from build123d import *

# Parameters (mm, degrees)
F0_W     = 44
F0_H     = 55
F2_R     = 20
F3_DEPTH = 133.830428
F4_W     = 29.281278
F4_H     = 21.154624
F5_DEPTH = 25


with BuildPart() as f1:
    # F0 (on Front) → F1 (revolve)
    with BuildSketch(Plane.XZ):
        with Locations((-22, 27.5)):
            Rectangle(F0_W, F0_H)
    revolve(axis=Axis((0, 0, 27.5), (0, 0, -1)))

    # F2 (on face) → F3 (cut)
    with BuildSketch(Plane(origin=(0, 0, 0), x_dir=(1, 0, 0), z_dir=(0, 0, -1))):
        with Locations((0, -15.39881)):
            Circle(F2_R)
    extrude(amount=-F3_DEPTH, mode=Mode.SUBTRACT)

    # F4 (on face) → F5 (cut)
    with BuildSketch(Plane.XY.offset(55)):
        with Locations((6.999669, -21.173684)):
            Rectangle(F4_W, F4_H)
    extrude(amount=-F5_DEPTH, mode=Mode.SUBTRACT)


solid = f1.part
Geometry check sheet. Reference: the model listing, model coordinates, mm. A direction names the side the tool comes from. Round coordinates to 2 decimals unless told otherwise and drop trailing zeros. Write each loop counter-clockwise with the first axis right and the second up, starting at its lowest first coordinate (ties: lowest second). Pieces come first, ordered by that corner, then holes. Notation, with made-up numbers: (64.25, -11.75) -> (82.25, -11.75) arc R22 ccw to (82.25, 11.25) -> close; hole circle Ø6 at (-12.5, 2). An arc over 180 degrees is marked (long way). One line per item, written item: value. Start each with the question number.
(1) Cross-section at D-D, the plane y = 30. Record the cut outline in (x, z), and give its area (3 significant figures).
(2) Cross-section at B-B, the plane x = 0. Record the cut outline in (y, z), and give its area (3 significant figures).
(3) Cross-section at A-A, the plane y = 0. Record the cut outline in (x, z).
(4) Cross-section at C-C, the plane z = 32. Record the cut outline in (x, y).
(5) Draft check along X on faces 1 (the cylindrical face through (10.752, -1.465, 27.115)), 2 (the cylindrical face through (9.538, -42.954, 27.885)), 3 (the flat face through (1, -9, 0)). Enter one of: +X half, -X half, draft (parallel to the pull), parting line (faces both ways), or undercut.
(6) Access from +Z, -Z, +X, -X, +Y, -Y to the whole of each face (thin tool, end or side, straight path). Record for faces 4 (the flat face through (1, -9, 55)), 5 (the flat face through (7, -21, 30)).
(7) Scan lines: line 1 (Y direction, x = 0, z = 40.5); line 2 (Y direction, x = 0, z = 29); line 3 (Y direction, x = 6, z = 30.5). Record each from-to range of solid material in increasing order. Write a range as [from, to].
(8) Go/stop test with flat-tipped pins: pin 1 Ø23.5 at (y, z) = (-18.5, 46) entering from +X; pin 2 Ø6 at (x, y) = (34, -21.5) entering from -Z; pin 3 Ø10 at (x, y) = (12.5, 22.5) entering from +Z; pin 4 Ø2 at (y, z) = (-33, 46) entering from -X. Record where each tip stops, or that it passes through.
Answer:
1. outline: (-32.19, 0) -> (-13.67, 0) -> (-13.67, 55) -> (-32.19, 55) -> close; (13.67, 0) -> (32.19, 0) -> (32.19, 55) -> (13.67, 55) -> close
1. area: 2,040 mm²
2. outline: (-44, 0) -> (-4.6, 0) -> (-4.6, 55) -> (-10.6, 55) -> (-10.6, 30) -> (-31.75, 30) -> (-31.75, 55) -> (-44, 55) -> close; (35.4, 0) -> (44, 0) -> (44, 55) -> (35.4, 55) -> close
2. area: 2,110 mm²
3. outline: (-44, 0) -> (-12.76, 0) -> (-12.76, 55) -> (-44, 55) -> close; (12.76, 0) -> (44, 0) -> (44, 55) -> (12.76, 55) -> close
4. outline: circle Ø88 at (0, 0); hole circle Ø40 at (0, 15.4); hole (-7.64, -31.75) -> (21.64, -31.75) -> (21.64, -10.6) -> (-7.64, -10.6) -> close
5. face 1: undercut
5. face 2: parting line
5. face 3: draft
6. face 4: +Z, +X, -X, +Y, -Y
6. face 5: +Z
7. line 1: [-44, -31.75], [-10.6, -4.6], [35.4, 44]
7. line 2: [-44, -4.6], [35.4, 44]
7. line 3: [-43.59, -31.75], [-10.6, -3.68], [34.48, 43.59]
8. pin 1: x = 43.48
8. pin 2: z = 0
8. pin 3: through
8. pin 4: x = -30.2
